Read the model definition and answer for the solid it produces. Units are mm, in the model's axes. Round coordinates to 2 decimals unless told otherwise and drop trailing zeros. Order: outer loops, then holes, each group sorted by start corner. A loop starts at its lowest first (then second) coordinate and runs counter-clockwise, first axis right, second up. Notation, with made-up numbers: (-20, 31) -> (2, 31) arc R9 ccw to (2, 39) -> close; hole circle Ø10 at (77, 20). An arc over 180 degrees is marked (long way). Answer as a JSON object with one key per item and string values. Group by question number.
Item 1: Consider probe 1 along Y at (x, z) = (-65, 2); probe 2 along X at (y, z) = (-1, 2.6); probe 3 along X at (y, z) = (31, 1.6). Determine where each line is inside the solid, lowest interval first. Write a range as from..to.
Item 2: The mould has two halves that part along X. Classify faces 1 (the flat face through (-34, 23, 0)), 2 (the cylindrical face through (37.04, -22.18, 1.48)), 3 (the flat face through (75, -1, 1)): pulls with the +X half, pulls with the -X half, needs draft (parallel to the pull), parting line crosses it, or undercut.
Item 3: Section D-D, the plane y = -44.5 is taken. Write down the section's boundary in (x, z), plus the area to 3 significant figures.
Item 4: Section A-A, the plane x = 42.5 is taken. Write down the section's boundary in (y, z), plus the area to 3 significant figures.
Item 5: Section C-C, the plane y = 0 is taken. Write down the section's boundary in (x, z), plus the area to 3 significant figures.
Item 6: Section B-B, the plane x = 0 is taken. Write down the section's boundary in (y, z).
from build123d import *

# Parameters (mm, degrees)
SKETCH_1_W      = 150
SKETCH_1_H      = 100
SKETCH_1_R      = 1.5
SKETCH_1_R_2    = 40
EXTRUDE_2_DEPTH = 3


with BuildPart() as part:
    # 草图1 → 凸台-拉伸2 (new body)
    with BuildSketch(Plane.XY):
        Rectangle(SKETCH_1_W, SKETCH_1_H)
        with Locations((-38.538130468, 22.25)):
            Circle(SKETCH_1_R, mode=Mode.SUBTRACT)
        with Locations((-38.538130468, -22.25)):
            Circle(SKETCH_1_R, mode=Mode.SUBTRACT)
        with Locations((0, -44.5)):
            Circle(SKETCH_1_R, mode=Mode.SUBTRACT)
        with Locations((38.538130468, -22.25)):
            Circle(SKETCH_1_R, mode=Mode.SUBTRACT)
        with Locations((38.538130468, 22.25)):
            Circle(SKETCH_1_R, mode=Mode.SUBTRACT)
        with Locations((0, 44.5)):
            Circle(SKETCH_1_R, mode=Mode.SUBTRACT)
        with Locations((-42.5, 0)):
            Circle(SKETCH_1_R, mode=Mode.SUBTRACT)
        with Locations((42.5, 0)):
            Circle(SKETCH_1_R, mode=Mode.SUBTRACT)
        Circle(SKETCH_1_R_2, mode=Mode.SUBTRACT)
        with Locations((65, 10)):
            Circle(SKETCH_1_R, mode=Mode.SUBTRACT)
        with Locations((65, -30)):
            Circle(SKETCH_1_R, mode=Mode.SUBTRACT)
        with Locations((-65, -30)):
            Circle(SKETCH_1_R, mode=Mode.SUBTRACT)
        with Locations((-65, -10)):
            Circle(SKETCH_1_R, mode=Mode.SUBTRACT)
        with Locations((-65, 10)):
            Circle(SKETCH_1_R, mode=Mode.SUBTRACT)
        with Locations((-65, 30)):
            Circle(SKETCH_1_R, mode=Mode.SUBTRACT)
        with Locations((65, -10)):
            Circle(SKETCH_1_R, mode=Mode.SUBTRACT)
        with Locations((65, 30)):
            Circle(SKETCH_1_R, mode=Mode.SUBTRACT)
    extrude(amount=EXTRUDE_2_DEPTH)


solid = part.part
Values found:
{
 "1": {"probe 1": "-50..-31.5, -28.5..-11.5, -8.5..8.5, 11.5..28.5, 31.5..50", "probe 2": "-75..-43.62, -41.38..-39.99, 39.99..41.38, 43.62..75", "probe 3": "-75..-66.12, -63.88..-25.28, 25.28..63.88, 66.12..75"},
 "2": {"face 1": "needs draft", "face 2": "undercut", "face 3": "pulls with the +X half"},
 "3": {"outline": "(-75, 0) -> (-1.5, 0) -> (-1.5, 3) -> (-75, 3) -> close; (1.5, 0) -> (75, 0) -> (75, 3) -> (1.5, 3) -> close", "area": "441 mm2"},
 "4": {"outline": "(-50, 0) -> (-1.5, 0) -> (-1.5, 3) -> (-50, 3) -> close; (1.5, 0) -> (50, 0) -> (50, 3) -> (1.5, 3) -> close", "area": "291 mm2"},
 "5": {"outline": "(-75, 0) -> (-44, 0) -> (-44, 3) -> (-75, 3) -> close; (-41, 0) -> (-40, 0) -> (-40, 3) -> (-41, 3) -> close; (40, 0) -> (41, 0) -> (41, 3) -> (40, 3) -> close; (44, 0) -> (75, 0) -> (75, 3) -> (44, 3) -> close", "area": "192 mm2"},
 "6": {"outline": "(-50, 0) -> (-46, 0) -> (-46, 3) -> (-50, 3) -> close; (-43, 0) -> (-40, 0) -> (-40, 3) -> (-43, 3) -> close; (40, 0) -> (43, 0) -> (43, 3) -> (40, 3) -> close; (46, 0) -> (50, 0) -> (50, 3) -> (46, 3) -> close"}
}
